Geometry check sheet. Reference: the model listing, model coordinates, mm. A direction names the side the tool comes from. Give positions to 0.01 mm unless a question says otherwise; leave off trailing zeros. Order: outer loops, then holes, each group sorted by start corner. A loop starts at its lowest first (then second) coordinate and runs counter-clockwise, first axis right, second up. Notation, with made-up numbers: M 71.5,65.5 L 126.5,65.5 A9 cw 126.5,79.5 Z; hole C 81.5,-13 d8. An arc over 180 degrees is marked long. Answer as CSV lines item,"result". Start each with the question number.
Q1. Go/stop test with flat-tipped pins: pin 1 (4 mm diameter, centred on x = 3, z = -1, fed in from -Y); pin 2 (2.5 mm diameter, centred on x = 8, y = -1, fed in from -Z); pin 3 (3 mm diameter, centred on x = -7, z = 41.5, fed in from +Y) (3 decimals); pin 4 (1 mm diameter, centred on x = -5, z = -9.5, fed in from -Y). Record where each tip stops, or that it passes through.
Q2. Thickness scan on line 1 (Z direction, x = -2, y = -7.75); line 2 (Y direction, x = 0.5, z = 53); line 3 (Y direction, x = 0.5, z = 29.5). Record the ranges inside material, lowest first.
Q3. Section check B-B, the plane x = 0. Record the boundary of the cut face in (y, z).
Q4. Set-up check for faces 1 (the flat face through (0.1, 10.2, 35)), 2 (the flat face through (-4, -6, 52)), 3 (the flat face through (2.7, 9.3, 45)): record each of +Z, -Z, +X, -X, +Y, -Y from which the full face is reachable in a straight line by a thin tool's end or side.
Q5. Mould release check, pull along Y, two halves, no side actions. Record for faces 4 (the flat face through (0, 0, 65)), 5 (the flat face through (9, 0, -45)), 6 (the cylindrical face through (4.38, -8.43, 48.55)): +Y half, -Y half, draft (parallel to the pull), parting line (faces both ways), or undercut.
Q6. Section check D-D, the plane z = -53. Record the boundary of the cut face in (x, y), then the cut area to 3 significant figures.
Q7. Section check C-C, the plane z = 28. Record the boundary of the cut face in (x, y).
Q8. Section check A-A, the plane y = 0. Record the boundary of the cut face in (x, z), then the cut area to 3 significant figures.
```python
from build123d import *

# Parameters (mm, degrees)
IZIM1_R                     = 12.5
Y_KSEKLIK_EKSTR_ZYON1_DEPTH = 65
IZIM2_R                     = 12.5
IZIM2_R_2                   = 10
KES_EKSTR_ZYON1_DEPTH       = 100
IZIM3_W                     = 20
IZIM3_H                     = 6
KES_EKSTR_ZYON2_DEPTH       = 3
IZIM4_R                     = 12.5
IZIM4_R_2                   = 9.5
KES_EKSTR_ZYON3_DEPTH       = 7
IZIM5_R                     = 12.5
IZIM5_R_2                   = 7
KES_EKSTR_ZYON4_DEPTH       = 6
IZIM6_R                     = 12.5
IZIM6_R_2                   = 9.5
KES_EKSTR_ZYON5_DEPTH       = 7


with BuildPart() as part:
    # Çizim1 → Yükseklik-Ekstrüzyon1 (new body, symmetric)
    with BuildSketch(Plane.XY):
        Circle(IZIM1_R)
    extrude(amount=Y_KSEKLIK_EKSTR_ZYON1_DEPTH, both=True)

    # Çizim2 → Kes-Ekstrüzyon1 (cut)
    with BuildSketch(Plane(origin=(0, 0, -65), x_dir=(-1, 0, 0), z_dir=(0, 0, -1))):
        Circle(IZIM2_R)
        Circle(IZIM2_R_2, mode=Mode.SUBTRACT)
    extrude(amount=-KES_EKSTR_ZYON1_DEPTH, mode=Mode.SUBTRACT)

    # Çizim3 → Kes-Ekstrüzyon2 (cut)
    with BuildSketch(Plane(origin=(10, 0, 0), x_dir=(0, 0, -1), z_dir=(1, 0, 0))):
        with Locations((55, 0)):
            Rectangle(IZIM3_W, IZIM3_H)
    extrude(amount=-KES_EKSTR_ZYON2_DEPTH, mode=Mode.SUBTRACT)

    # Çizim4 → Kes-Ekstrüzyon3 (cut)
    with BuildSketch(Plane.XY.offset(65)):
        Circle(IZIM4_R)
        Circle(IZIM4_R_2, mode=Mode.SUBTRACT)
    extrude(amount=-KES_EKSTR_ZYON3_DEPTH, mode=Mode.SUBTRACT)

    # Çizim5 → Kes-Ekstrüzyon4 (cut)
    with BuildSketch(Plane.XY.offset(58)):
        Circle(IZIM5_R)
        Circle(IZIM5_R_2, mode=Mode.SUBTRACT)
    extrude(amount=-KES_EKSTR_ZYON4_DEPTH, mode=Mode.SUBTRACT)

    # Çizim6 → Kes-Ekstrüzyon5 (cut)
    with BuildSketch(Plane.XY.offset(52)):
        Circle(IZIM6_R)
        Circle(IZIM6_R_2, mode=Mode.SUBTRACT)
    extrude(amount=-KES_EKSTR_ZYON5_DEPTH, mode=Mode.SUBTRACT)


solid = part.part
```
Answer block:
1,pin 1,"stops at y = -9.95"
1,pin 2,"stops at z = -65"
1,pin 3,"stops at y = 11.225"
1,pin 4,"stops at y = -8.93"
2,line 1,"z = -65 to 52, 58 to 65"
2,line 2,"y = -6.98 to 6.98"
2,line 3,"y = -9.99 to 9.99"
3,outline,"M -12.5,35 L -10,35 L -10,-65 L 10,-65 L 10,35 L 12.5,35 L 12.5,45 L 9.5,45 L 9.5,52 L 7,52 L 7,58 L 9.5,58 L 9.5,65 L -9.5,65 L -9.5,58 L -7,58 L -7,52 L -9.5,52 L -9.5,45 L -12.5,45 Z"
4,face 1,"-Z"
4,face 2,"none"
4,face 3,"+Z"
5,face 4,"draft"
5,face 5,"undercut"
5,face 6,"parting line"
6,outline,"M 7,-3 L 7,3 L 9.54,3 A10 ccw long 9.54,-3 Z"
6,area,"297 mm2"
7,outline,"C 0,0 d20"
8,outline,"M -12.5,35 L -10,35 L -10,-65 L 7,-65 L 7,-45 L 10,-45 L 10,35 L 12.5,35 L 12.5,45 L 9.5,45 L 9.5,52 L 7,52 L 7,58 L 9.5,58 L 9.5,65 L -9.5,65 L -9.5,58 L -7,58 L -7,52 L -9.5,52 L -9.5,45 L -12.5,45 Z"
8,area,"2,540 mm2"
